Geometry: final body of the model. Coordinates: model frame, mm. A direction names the side the tool comes from. Round coordinates to 2 decimals unless told otherwise and drop trailing zeros. Loops run counter-clockwise (first coordinate to the right, second up) from the corner with the lowest first, then second, coordinate; pieces in that order, holes last. Notation, with made-up numbers: (89, 60) -> (109, 60) arc R18 cw to (109, 73) -> close; hole circle Ø8 at (-21.75, 80). An arc over 180 degrees is marked (long way). Answer in a Markdown table with one row per item.
Autodesk Inventor part; units mm, degrees
ref_plane "YZ Plane" through (0, 0, 0) normal (1, 0, 0) x (0, 1, 0)
ref_plane "XZ Plane" through (0, 0, 0) normal (0, 1, 0) x (-1, 0, 0)
ref_plane "XY Plane" through (0, 0, 0) normal (0, 0, 1) x (1, 0, 0)
sketch "Эскиз1" plane through (0, 0, 0) normal (0, 1, 0) x (-1, 0, 0)
  line L0 (-35, 57.5) -> (35, 57.5)
  line L1 (35, 57.5) -> (35, -57.5)
  line L2 (35, -57.5) -> (-35, -57.5)
  line L3 (-35, -57.5) -> (-35, 57.5)
  line L4 (-35, 57.5) -> (35, -57.5) construction
  line L5 (35, 57.5) -> (-35, -57.5) construction
  point P0 (0, 0)
  dimension "d0" = 115
  dimension "d1" = 70
extrude "Выдавливание1" add sketch "Эскиз1" along normal blind 4
sketch "Эскиз2" plane through (0, 4, 0) normal (0, 1, 0) x (1, 0, 0)
  line L0 (35, 57.5) -> (-35, 57.5)
  line L1 (35, -57.5) -> (-35, -57.5)
  line L2 (-35, -57.5) -> (-35, 57.5)
  line L3 (-35, 57.5) -> (35, 57.5)
  line L4 (35, 57.5) -> (35, -57.5)
  line L5 (35, -57.5) -> (-35, 57.5) construction
  line L6 (-35, -57.5) -> (35, 57.5) construction
  line L7 (31, -53.5) -> (-31, -53.5)
  line L8 (-31, -53.5) -> (-31, 53.5)
  line L9 (-31, 53.5) -> (31, 53.5)
  line L10 (31, 53.5) -> (31, -53.5)
  line L11 (31, -53.5) -> (-31, 53.5) construction
  line L12 (-31, -53.5) -> (31, 53.5) construction
  point P0 (0, 0)
  dimension "d4" = 4
  dimension "d5" = 4
extrude "Выдавливание2" add sketch "Эскиз2" along normal blind 64
sketch "Эскиз3" plane through (35, 0, 57.5) normal (1, 0, 0) x (0, 0, -1)
  line L0 (111, 4) -> (4, 4)
  line L1 (15, 4) -> (55, 4)
  line L2 (55, 4) -> (55, 27)
  line L3 (55, 27) -> (15, 27)
  line L4 (15, 27) -> (15, 4)
  point P0 (57.5, 0)
  point P1 (0, 0)
  dimension "d9" = 40
  dimension "d10" = 23
extrude "Выдавливание3" cut sketch "Эскиз3" against normal blind 75
sketch "Эскиз4" plane through (35, 0, 57.5) normal (1, 0, 0) x (0, 0, -1)
  line L0 (55, 27) -> (55, 4)
  circle A0 centre (99, 15.5) radius 1.5
  point P0 (57.5, 0)
  dimension "d14" = 3
extrude "Выдавливание4" cut sketch "Эскиз4" against normal blind 75
sketch "Эскиз5" plane through (-31, 4, -53.5) normal (1, 0, 0) x (0, 0, -1)
  line L0 (-107, 0) -> (-107, 64)
  line L1 (-107, 64) -> (-49.5, 64)
  line L2 (-49.5, 64) -> (-49.5, 35.4088)
  line L3 (-49.5, 35.4088) -> (-53.5, 35.4088)
  line L4 (-53.5, 35.4088) -> (-53.5, 60)
  line L5 (-53.5, 60) -> (-107, 60)
  line L6 (-107, 60) -> (-107, 64)
  point P0 (-53.5, -4)
  dimension "d17" = 4
  dimension "d18" = 4
extrude "Выдавливание5" add sketch "Эскиз5" along normal blind 62
sketch "Эскиз6" plane through (0, 0, 0) normal (0, -1, 0) x (1, 0, 0)
  line L0 (-20.5745, 51.4953) -> (20.4255, 51.4953)
  line L1 (20.4255, 51.4953) -> (20.4255, 46.4953)
  line L2 (20.4255, 46.4953) -> (-20.5745, 46.4953)
  line L3 (-20.5745, 46.4953) -> (-20.5745, 51.4953)
  line L4 (-20.5745, 51.4953) -> (20.4255, 46.4953) construction
  line L5 (20.4255, 51.4953) -> (-20.5745, 46.4953) construction
  point P0 (0, 0)
  point P1 (-0.0745, 48.9953)
  dimension "d21" = 5
  dimension "d22" = 41
extrude "Выдавливание6" cut sketch "Эскиз6" against normal blind 10
properties part number "самосвал кузов"
Item 1: Cut plane B-B (y = 15.5). Output: boundary loops of the cut face in (x, z).
Answer:
| item | result |
|---|---|
| outline | (-35, -57.5) -> (35, -57.5) -> (35, -43) -> (31, -43) -> (31, -53.5) -> (-31, -53.5) -> (-31, -43) -> (-35, -43) -> close; (-35, -40) -> (-31, -40) -> (-31, 2.5) -> (-35, 2.5) -> close; (-35, 42.5) -> (-31, 42.5) -> (-31, 53.5) -> (31, 53.5) -> (31, 42.5) -> (35, 42.5) -> (35, 57.5) -> (-35, 57.5) -> close; (31, -40) -> (35, -40) -> (35, 2.5) -> (31, 2.5) -> close |
Item 2: Cut plane C-C (x = -29.5). Output: boundary loops of the cut face in (y, z), then the cut area to 3 significant figures.
Answer:
| item | result |
|---|---|
| outline | (0, -57.5) -> (68, -57.5) -> (68, -53.5) -> (4, -53.5) -> (4, 53.5) -> (64, 53.5) -> (64, 0) -> (39.41, 0) -> (39.41, -4) -> (68, -4) -> (68, 57.5) -> (0, 57.5) -> close |
| area | 1,300 mm² |
Item 3: Pin query (flat end, axial travel): pin 1 Ø4.5 at (x, z) = (-33, 29) entering from -Y; pin 2 Ø1.5 at (x, z) = (-16.5, -20.5) entering from +Y. Return the tip coordinate at first contact, or that it passes through.
Answer:
| item | result |
|---|---|
| pin 1 | stops at y = 0 |
| pin 2 | stops at y = 4 |
Item 4: Line query: probe 1 along Z at (x, y) = (7, 45); probe 2 along Y at (x, z) = (-24.5, 10.5); probe 3 along X at (y, z) = (34, 36). Output: solid intervals per line, ascending. Write a range as [from, to].
Answer:
| item | result |
|---|---|
| probe 1 | z = [-57.5, -53.5], [-4, 0], [53.5, 57.5] |
| probe 2 | y = [0, 4], [64, 68] |
| probe 3 | x = [-35, -31], [31, 35] |
Item 5: Reachability of faces 4 (the face through (-33, 15, 2.5)), 5 (the face through (0, 34, 53.5)), 6 (the face through (0, 36, -53.5)), 7 (the face through (-35, 34, 1)), 8 (the face through (0, 2, 46.495)) from +Z, -Z, +X, -X, +Y, -Y: full face, straight path, thin tool, end or side. Return the list, or none.
Answer:
| item | result |
|---|---|
| face 4 | +X, -X |
| face 5 | none |
| face 6 | +Y |
| face 7 | +Z, -Z, -X, +Y, -Y |
| face 8 | -Y |
Item 6: Cut plane D-D (z = 10). Output: boundary loops of the cut face in (x, y), then the cut area to 3 significant figures.
Answer:
| item | result |
|---|---|
| outline | (-35, 0) -> (35, 0) -> (35, 4) -> (-35, 4) -> close; (-35, 27) -> (-31, 27) -> (-31, 64) -> (31, 64) -> (31, 27) -> (35, 27) -> (35, 68) -> (-35, 68) -> close |
| area | 856 mm² |
Item 7: Draft query along Z for faces 1 (the face through (0, 34, -57.5)), 2 (the face through (0, 4, -1)), 3 (the face through (35, 34, -1)). Return one class per face: pulls with the +Z half, pulls with the -Z half, needs draft (parallel to the pull), parting line crosses it, or undercut.
Answer:
| item | result |
|---|---|
| face 1 | pulls with the -Z half |
| face 2 | undercut |
| face 3 | needs draft |
Item 8: Cut plane A-A (z = -41.5). Output: boundary loops of the cut face in (x, y).
Answer:
| item | result |
|---|---|
| outline | (-35, 0) -> (35, 0) -> (35, 14) -> (31, 14) -> (31, 4) -> (-31, 4) -> (-31, 14) -> (-35, 14) -> close; (-35, 17) -> (-31, 17) -> (-31, 68) -> (-35, 68) -> close; (31, 17) -> (35, 17) -> (35, 68) -> (31, 68) -> close |
